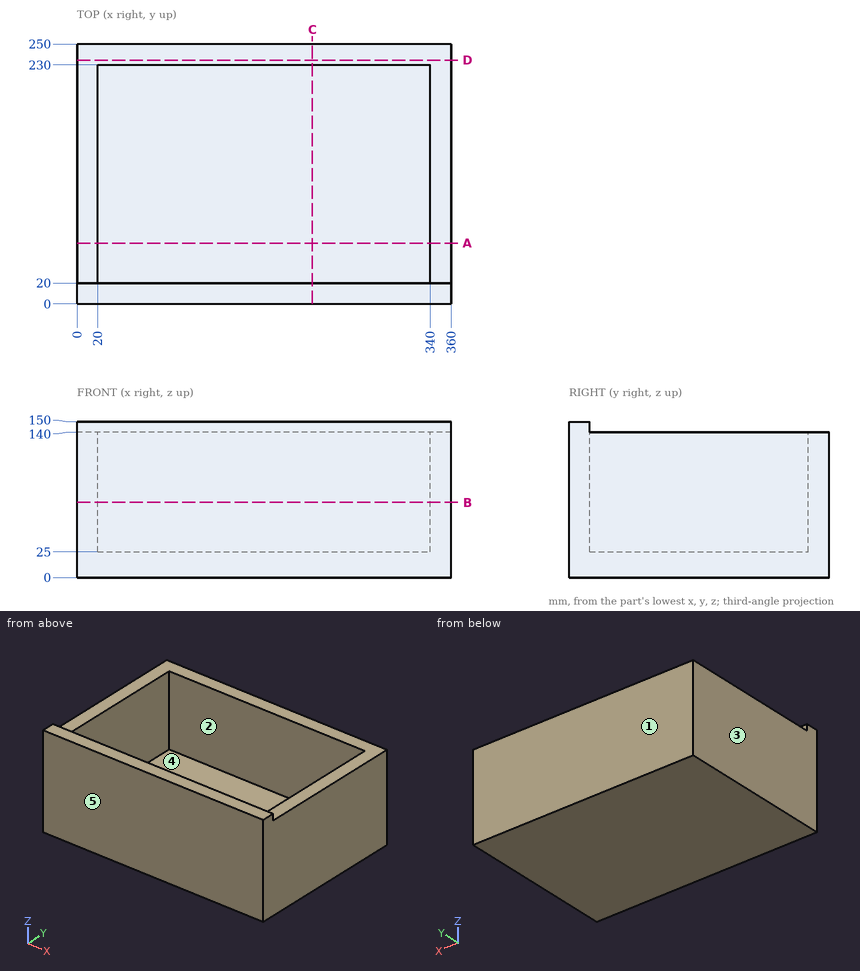
Could you check a few things on this drawing? It's one solid part, dimensions in mm from its lowest x, y, z. A direction names the side the tool comes from. Coordinates: 2 decimals unless noted, no trailing zeros. Loops run counter-clockwise (first coordinate to the right, second up) from the corner with the lowest first, then second, coordinate; pieces in that order, holes last. Notation, with made-up numbers: (-34.75, -11) - (6.25, -11) arc R28 ccw to (6.25, 7) - close; hole circle Ø7 at (54, -8). An arc over 180 degrees is marked (long way). Return JSON: item names as keys, results as strings. Group by question number.
Item 1: If we section it at D-D on y = 234.5: Write out the boundary of the cut face in (x, z).
Item 2: If we section it at C-C on x = 226.5: Write out the boundary of the cut face in (y, z).
Item 3: We'd pull the mould along X, two halves only. Please class the marked faces 1, 2 and 3: +X half, -X half, draft (parallel to the pull), parting line (faces both ways), or undercut.
Item 4: Will this pin go through, and if not, where does the flat tip stop? P1, Ø4, axis at x = 261, y = 106, coming from the +Z side.
Item 5: On a 3-axis mill with a long thin cutter (end or side, diameter ignored), from which of +Z, -Z, +X, -X, +Y, -Y can I reach the whole of each face in a straight line? I mean the marked faces 4 and 5. Say none if no direction works.
Item 6: If we section it at A-A on y = 58.5: Write out the boundary of the cut face in (x, z), and give its area (3 significant figures).
Item 7: I need wall thicknesses on line 1 (Y direction, x = 26.5, z = 46.5); line 2 (X direction, y = 221, z = 81); line 3 (Z direction, x = 117.5, y = 109). Which ranges of each line are inside material? Lowest first, please. Write a range as from..to.
Item 8: If we section it at B-B on z = 72.5: Write out the boundary of the cut face in (x, y), and give its area (3 significant figures).
Calculated:
{
 "1": {"outline": "(0, 0) - (360, 0) - (360, 140) - (0, 140) - close"},
 "2": {"outline": "(0, 0) - (250, 0) - (250, 140) - (230, 140) - (230, 25) - (20, 25) - (20, 150) - (0, 150) - close"},
 "3": {"face 1": "draft", "face 2": "undercut", "face 3": "-X half"},
 "4": {"P1": "stops at z = 25"},
 "5": {"face 4": "+Z", "face 5": "+Z, -Z, +X, -X, -Y"},
 "6": {"outline": "(0, 0) - (360, 0) - (360, 140) - (340, 140) - (340, 25) - (20, 25) - (20, 140) - (0, 140) - close", "area": "13,600 mm^2"},
 "7": {"line 1": "y = 0..20, 230..250", "line 2": "x = 0..20, 340..360", "line 3": "z = 0..25"},
 "8": {"outline": "(0, 0) - (360, 0) - (360, 250) - (0, 250) - close; hole (20, 20) - (340, 20) - (340, 230) - (20, 230) - close", "area": "22,800 mm^2"}
}
